Job drawing, mm, ordinate dimensions from the low corner. One solid piece. A direction names the side the tool comes from. Give positions to 0.01 mm unless a question says otherwise; leave off trailing zeros. Order: outer loops, then holes, each group sorted by start corner. A loop starts at its lowest first (then second) coordinate and runs counter-clockwise, first axis right, second up. Notation, with made-up numbers: (59.25, 59) - (100.25, 59) arc R33 cw to (100.25, 95) - close; hole circle Ø4 at (25, -24). An arc over 180 degrees is marked (long way). Write each question's results on one line, items separated by ' | '. Start each with the question number.
1) Cut at A-A on x = 14.5. List the corners of the cut face in (y, z), plus the area to 3 significant figures.
2) Two-plate mould, pull along X, no slides. Class the marked faces 3, 4, 5 and 6: +X half, -X half, draft (parallel to the pull), parting line (faces both ways), or undercut.
3) Drill centre lines: line 1 along Y through (x, z) = (14.5, 8); line 2 along Y through (x, z) = (14.5, 1.55); line 3 along Z through (x, y) = (13.5, 2.5). Where is each one in solid material? Low to high. Write a range as from..to.
4) Drop flat-ended pins along their axis: pin 1 Ø8 at (x, y) = (19, 13) entering from +Z; pin 2 Ø5 at (x, z) = (24.5, 1) entering from -Y. Give the stop position or say it passes through.
5) Tool access for the marked faces 1 and 2: list every direction of +Z, -Z, +X, -X, +Y, -Y with a clear straight run to the whole face (end or side of a thin tool).
6) Cut at D-D on x = 26.75. List the corners of the cut face in (y, z).
7) Cut at C-C on y = 10. List the corners of the cut face in (x, z).
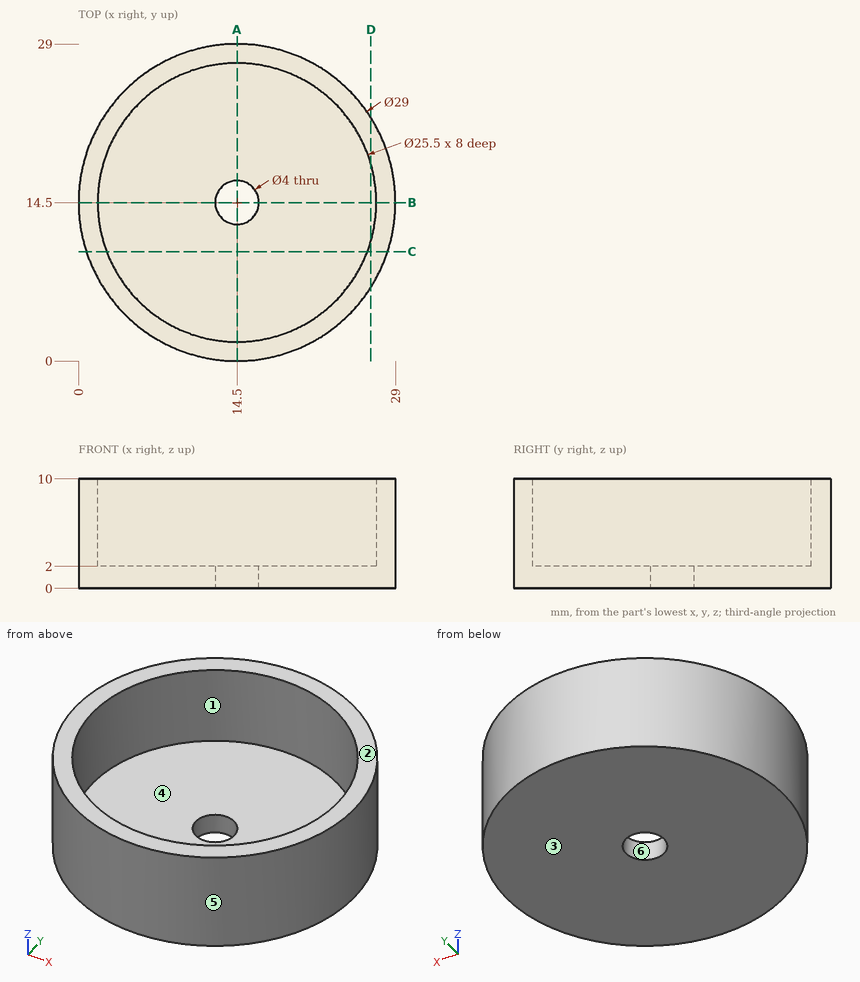
Results:
1) outline: (0, 0) - (12.5, 0) - (12.5, 2) - (1.75, 2) - (1.75, 10) - (0, 10) - close; (16.5, 0) - (29, 0) - (29, 10) - (27.25, 10) - (27.25, 2) - (16.5, 2) - close | area: 78.0 mm^2
2) face 3: draft | face 4: undercut | face 5: parting line | face 6: undercut
3) line 1: 0..1.75, 27.25..29 | line 2: 0..12.5, 16.5..29 | line 3: 0..2
4) pin 1: z = 2 | pin 2: y = 2.09
5) face 1: +Z | face 2: +Z, +X, -X, +Y, -Y
6) outline: (6.74, 0) - (22.26, 0) - (22.26, 10) - (18.04, 10) - (18.04, 2) - (10.96, 2) - (10.96, 10) - (6.74, 10) - close
7) outline: (0.72, 0) - (28.28, 0) - (28.28, 10) - (26.43, 10) - (26.43, 2) - (2.57, 2) - (2.57, 10) - (0.72, 10) - close
